Autodesk Inventor part; units mm, degrees
ref_plane "YZ Plane" through (0, 0, 0) normal (1, 0, 0) x (0, 1, 0)
ref_plane "XZ Plane" through (0, 0, 0) normal (0, 1, 0) x (-1, 0, 0)
ref_plane "XY Plane" through (0, 0, 0) normal (0, 0, 1) x (1, 0, 0)
sketch "Sketch1" plane through (0, 0, 0) normal (0, 1, 0) x (-1, 0, 0)
  line L0 (3.7528, 6.5) -> (7.5056, 0)
  line L1 (7.5056, 0) -> (3.7528, -6.5)
  line L2 (3.7528, -6.5) -> (-3.7528, -6.5)
  line L3 (-3.7528, -6.5) -> (-7.5056, 0)
  line L4 (-7.5056, 0) -> (-3.7528, 6.5)
  line L5 (-3.7528, 6.5) -> (3.7528, 6.5)
  point P0 (0, 0)
  point P1 (0, 0)
  dimension "d0" = 6.5
extrude "Extrusion1" add sketch "Sketch1" along normal blind 6.5
sketch "Sketch2" plane through (0, 6.5, 0) normal (0, 1, 0) x (1, 0, 0)
  point P0 (0, 0)
hole "Hole1" at (0, 6.5, 0) direction (0, -1, 0) diameter 6.647 depth 8 tip angle 118
sketch "Sketch3" plane through (0, 6.5, 0) normal (0, 1, 0) x (1, 0, 0)
  circle A0 centre (0, 0) radius 3.3235
  circle A1 centre (0, 0) radius 6.5
  circle A2 centre (0, 0) radius 29.8584
extrude "Extrusion2" cut sketch "Sketch3" against normal blind 1 draft -60 contours A2
sketch "Sketch4" plane through (0, 0, 0) normal (0, -1, 0) x (1, 0, 0)
  circle A0 centre (0, 0) radius 3.3235
  circle A1 centre (0, 0) radius 6.5
  circle A2 centre (0, 0) radius 18
extrude "Extrusion3" cut sketch "Sketch4" against normal blind 1 draft -60 contours A2
fillet "Fillet1" radius 0.5 6 edges at (-7.5056, 3.25, 0) (-3.7528, 3.25, 6.5) (3.7528, 3.25, 6.5) (7.5056, 3.25, 0) (3.7528, 3.25, -6.5) (-3.7528, 3.25, -6.5)
chamfer "Chamfer1" distance 0.5 angle 45 2 edges at (0, 6.5, -3.3235) (0, 0, -3.3235)
properties part number "bed nut" material "Stainless Steel"
CAD build for the part. Positions are in the model's coordinates, mm. Coordinates: 2 decimals unless noted, no trailing zeros. Write each loop counter-clockwise with the first axis right and the second up, starting at its lowest first coordinate (ties: lowest second). Pieces come first, ordered by that corner, then holes. Notation, with made-up numbers: (13, 57.5) - (69, 57.5) arc R5 cw to (69, 62.5) - close; hole circle Ø1 at (47.5, 17.25). An arc over 180 degrees is marked (long way). Use a Markdown table: item, result. Add a question column.
Item 1: Band-saw the part on A-A, the plane z = 0. Give the cut face in (x, y).
Item 2: Band-saw the part on B-B, the plane y = 2.75. Give the cut face in (x, z).
Item 3: Mould opens along Z. For faces 1 (the face through (5.65, 3.2, 3.21)), 2 (the face through (-3.39, 6.35, -5.85)), 3 (the face through (1.27, 3.21, 3.07)) say: pulls with the +Z half, pulls with the -Z half, needs draft (parallel to the pull), parting line crosses it, or undercut.
Item 4: Drill centre lines: L1, parallel to X at y = 3.95, z = 0; L2, parallel to Z at x = 0, y = 2.1; L3, parallel to X at y = 1.5, z = 0.5. Where is each one in solid material? Low to high. Write a range as from..to.
Numbers:
| question | item | result |
|---|---|---|
| 1 | outline | (-7.43, 0.54) - (-6.5, 0) - (-3.82, 0) - (-3.32, 0.5) - (-3.32, 6) - (-3.82, 6.5) - (-6.5, 6.5) - (-7.43, 5.96) - close; (3.32, 0.5) - (3.82, 0) - (6.5, 0) - (7.43, 0.54) - (7.43, 5.96) - (6.5, 6.5) - (3.82, 6.5) - (3.32, 6) - close |
| 2 | outline | (-7.36, -0.25) - (-3.9, -6.25) arc R0.5 ccw to (-3.46, -6.5) - (3.46, -6.5) arc R0.5 ccw to (3.9, -6.25) - (7.36, -0.25) arc R0.5 ccw to (7.36, 0.25) - (3.9, 6.25) arc R0.5 ccw to (3.46, 6.5) - (-3.46, 6.5) arc R0.5 ccw to (-3.9, 6.25) - (-7.36, 0.25) arc R0.5 ccw to start; hole circle Ø6.65 at (0, 0) |
| 3 | face 1 | pulls with the +Z half |
| 3 | face 2 | pulls with the -Z half |
| 3 | face 3 | undercut |
| 4 | L1 | -7.43..-3.32, 3.32..7.43 |
| 4 | L2 | -6.5..-3.32, 3.32..6.5 |
| 4 | L3 | -7.22..-3.29, 3.29..7.22 |
